Input: part model. Units: mm. Frame: model coordinates. Give positions to 0.01 mm unless a question says otherwise; leave off trailing zeros. Loops run counter-clockwise (first coordinate to the right, second up) from the corner with the lowest first, then second, coordinate; pieces in that order, holes last. Notation, with made-up numbers: (24.25, 75) - (65.25, 75) arc R24 cw to (65.25, 87) - close; hole circle Ø6 at (80.5, -33.5). An arc over 180 degrees is marked (long way). Answer as a JSON object with one key per item and string values.
from build123d import *

# Parameters (mm, degrees)
SKETCH_1_W          = 95
SKETCH_1_H          = 33
EXTRUDE_1_DEPTH     = 3
SKETCH_2_R          = 1.5
CUT_EXTRUDE_1_DEPTH = 4
SKETCH_3_R          = 1.5
CUT_EXTRUDE_2_DEPTH = 4
FILLET_1_R          = 3
SKETCH_4_W          = 28.872486122
SKETCH_4_H          = 10.738590994
CUT_EXTRUDE_3_DEPTH = 4
FILLET_2_R          = 3


with BuildPart() as part:
    # 草图1 → 凸台-拉伸1 (new body)
    with BuildSketch(Plane(origin=(0, 0, 0), x_dir=(1, 0, 0), z_dir=(0, 1, 0))):
        Rectangle(SKETCH_1_W, SKETCH_1_H)
    extrude(amount=EXTRUDE_1_DEPTH)

    # 草图2 → 切除-拉伸1 (cut, through all)
    with BuildSketch(Plane(origin=(0, 3, 0), x_dir=(1, 0, 0), z_dir=(0, 1, 0))):
        with Locations((-44, 11.375)):
            Circle(SKETCH_2_R)
        with Locations((-44, -11.375)):
            Circle(SKETCH_2_R)
        with Locations((44, -11.375)):
            Circle(SKETCH_2_R)
        with Locations((44, 11.375)):
            Circle(SKETCH_2_R)
    extrude(amount=-CUT_EXTRUDE_1_DEPTH, mode=Mode.SUBTRACT)

    # 草图3 → 切除-拉伸2 (cut, through all)
    with BuildSketch(Plane(origin=(0, 3, 0), x_dir=(1, 0, 0), z_dir=(0, 1, 0))):
        with Locations((-24, 9)):
            Circle(SKETCH_3_R)
        with Locations((24, 9)):
            Circle(SKETCH_3_R)
        with Locations((-24, -9)):
            Circle(SKETCH_3_R)
        with Locations((24, -9)):
            Circle(SKETCH_3_R)
    extrude(amount=-CUT_EXTRUDE_2_DEPTH, mode=Mode.SUBTRACT)

    # 圆角1
    fillet_1_edges = [part.edges().sort_by_distance(p)[0] for p in [
        (-47.5, 1.5, -16.5),
        (47.5, 1.5, -16.5),
        (47.5, 1.5, 16.5),
        (-47.5, 1.5, 16.5),
    ]]
    fillet(fillet_1_edges, radius=FILLET_1_R)

    # 草图4 → 切除-拉伸3 (cut, through all)
    with BuildSketch(Plane(origin=(0, 3, 0), x_dir=(1, 0, 0), z_dir=(0, 1, 0))):
        Rectangle(SKETCH_4_W, SKETCH_4_H)
    extrude(amount=-CUT_EXTRUDE_3_DEPTH, mode=Mode.SUBTRACT)

    # 圆角2
    fillet_2_edges = [part.edges().sort_by_distance(p)[0] for p in [
        (-14.436243061, 1.5, 5.369295497),
        (-14.436243061, 1.5, -5.369295497),
        (14.436243061, 1.5, -5.369295497),
        (14.436243061, 1.5, 5.369295497),
    ]]
    fillet(fillet_2_edges, radius=FILLET_2_R)


solid = part.part
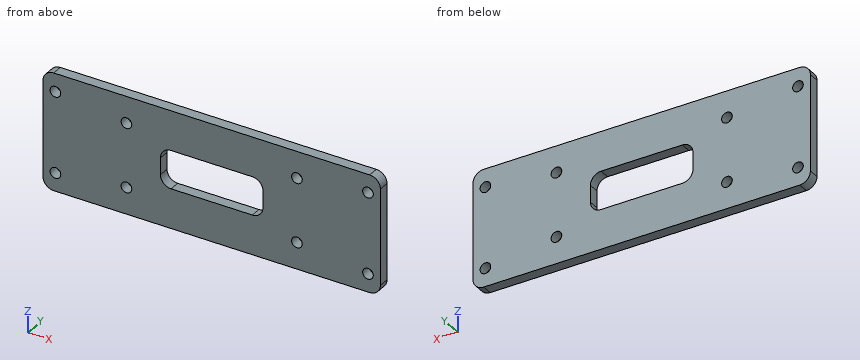
Item 1: Cut plane D-D (y = 2.2). Give the number of separate pieces and of enclosed holes in the cut face, then the cut area to 3 significant figures.
Geometry check:
{"separate pieces": "1", "enclosed holes": "9", "area": "2,770 mm2"}
Item 2: Cut plane B-B (z = -9). Return loops of the section in (x, y), then the cut area to 3 significant figures.
Geometry check:
{"outline": "(-47.5, 0) - (-25.5, 0) - (-25.5, 3) - (-47.5, 3) - close; (-22.5, 0) - (22.5, 0) - (22.5, 3) - (-22.5, 3) - close; (25.5, 0) - (47.5, 0) - (47.5, 3) - (25.5, 3) - close", "area": "267 mm2"}
Item 3: Cut plane A-A (x = 7). Return loops of the section in (y, z).
Geometry check:
{"outline": "(0, -16.5) - (3, -16.5) - (3, -5.37) - (0, -5.37) - close; (0, 5.37) - (3, 5.37) - (3, 16.5) - (0, 16.5) - close"}
Item 4: Cut plane C-C (z = 4). Return loops of the section in (x, y), then the cut area to 3 significant figures.
Geometry check:
{"outline": "(-47.5, 0) - (-13.95, 0) - (-13.95, 3) - (-47.5, 3) - close; (13.95, 0) - (47.5, 0) - (47.5, 3) - (13.95, 3) - close", "area": "201 mm2"}
Item 5: Material intervals for line 1 (X direction, y = 1, z = 9); line 2 (Z direction, x = -24, y = 0.45); line 3 (X direction, y = 2.1, z = -12), sorted ascending. Write a range as [from, to].
Geometry check:
{"line 1": "x = [-47.5, -25.5], [-22.5, 22.5], [25.5, 47.5]", "line 2": "z = [-16.5, -10.5], [-7.5, 7.5], [10.5, 16.5]", "line 3": "x = [-47.5, -45.36], [-42.64, 42.64], [45.36, 47.5]"}
